Part model, mm, in its own coordinate system. A direction names the side the tool comes from. Round coordinates to 2 decimals unless told otherwise and drop trailing zeros. Loops run counter-clockwise (first coordinate to the right, second up) from the corner with the lowest first, then second, coordinate; pieces in that order, holes last. Notation, with made-up numbers: M 80.5,-12.5 L 126.5,-12.5 A35 ccw 126.5,20.5 Z; hole C 84.25,45.5 d11. An arc over 180 degrees is marked long. Put each result on its own line as item: value. Start each with the question number.
1) Pull direction Z, two halves, no side cores. Call faces 4 (the flat face through (99, 5.08, 80)), 5 (the cylindrical face through (-14.32, 2.5, 157.6)), 6 (the cylindrical face through (-5.091, 2.504, 170.157)): +Z half, -Z half, draft (parallel to the pull), parting line (faces both ways), or undercut.
2) Drop flat-ended pins along their axis: pin 1 Ø5.5 at (x, z) = (21.7, 156.88) entering from +Y; pin 2 Ø1.5 at (x, y) = (164.5, 2) entering from +Z; pin 3 Ø2 at (x, y) = (-14.5, 2) entering from +Z; pin 4 Ø2 at (x, y) = (5.5, 3.5) entering from -Z. Give the stop position or say it passes through.
3) Probe line 1 along X through (y, z) = (0.75, 49); line 2 along X through (y, z) = (3.85, 107.5); line 3 along Z through (x, y) = (-3.5, 2.3). List the from-to ranges inside material, lowest first.
4) Slice it at C-C on z = 107.5. Give the cut face in (x, y).
5) Which spindle directions (+Z, -Z, +X, -X, +Y, -Y) get a long thin tool onto all of the face, cutting with end or side? Do faces 1 (the cylindrical face through (211.089, 2.576, 141.796)), 2 (the flat face through (209.902, 2.576, 24.426)), 3 (the flat face through (69.827, 2.576, 71.224)). Say none if no direction does.
6) Slice it at D-D on x = 148. Give the cut face in (y, z).
7) Slice it at A-A on x = 180. Give the cut face in (y, z), then the cut area to 3 significant figures.
8) Slice it at B-B on z = 54.5. Give the cut face in (x, y).
```python
from build123d import *

# Parameters (mm, degrees)
SKETCH3_R           = 2.5
SKETCH3_R_2         = 52.3875
SKETCH3_R_3         = 3.3
SKETCH3_R_4         = 4.5
SKETCH3_R_5         = 27.4955
SKETCH3_R_6         = 3.300000004
BOSS_EXTRUDE1_DEPTH = 5.08
CUT_EXTRUDE1_REACH  = 321.397
CUT_EXTRUDE2_REACH  = 321.397
CUT_EXTRUDE4_REACH  = 321.397
CUT_EXTRUDE5_REACH  = 321.397
CUT_EXTRUDE6_REACH  = 321.397
FILLET1_R           = 6.604


with BuildPart() as part:
    # Sketch3 → Boss-Extrude1 (new body)
    with BuildSketch(Plane(origin=(0, 0, 0), x_dir=(-1, 0, 0), z_dir=(0, 1, 0))):
        with BuildLine():
            Line((-47.164225852, 28.786858925), (1.714987837, 81.055723289))
            ThreePointArc((1.714987837, 81.055723289), (46.941307752, 112.338258021), (29.825562347, 164.597881552))
            ThreePointArc((29.825562347, 164.597881552), (28.145398332, 165.051242365), (26.567761736, 164.316701751))
            Line((26.567761736, 164.316701751), (21.302878118, 159.051818133))
            ThreePointArc((21.302878118, 159.051818133), (14.21924173, 157.642795249), (10.20668404, 163.648012211))
            Line((10.20668404, 163.648012211), (10.20668404, 170.220745001))
            ThreePointArc((10.20668404, 170.220745001), (9.549518747, 171.925600851), (7.91807501, 172.748273949))
            ThreePointArc((7.91807501, 172.748273949), (3.367898451, 172.974), (-1.182278109, 172.748273949))
            ThreePointArc((-1.182278109, 172.748273949), (-2.813721846, 171.925600851), (-3.470887139, 170.220745001))
            Line((-3.470887139, 170.220745001), (-3.470887139, 163.648012211))
            ThreePointArc((-3.470887139, 163.648012211), (-9.970887139, 157.148012211), (-16.470887139, 163.648012211))
            Line((-16.470887139, 163.648012211), (-16.470887139, 164.225022653))
            ThreePointArc((-16.470887139, 164.225022653), (-17.760387302, 166.435870942), (-20.319588051, 166.401924563))
            Line((-20.319588051, 166.401924563), (-168.403592651, 158.863977372))
            Line((-168.403592651, 158.863977372), (-265.178957518, 163.648012211))
            Line((-265.178957518, 163.648012211), (-268.446360693, 19.778758396))
            ThreePointArc((-268.446360693, 19.778758396), (-262.000922025, 10.329558641), (-251.128758127, 13.883022842))
            Line((-251.128758127, 13.883022842), (-65.147106167, 22.945506915))
            ThreePointArc((-65.147106167, 22.945506915), (-52.854167936, 15.702363891), (-47.164225852, 28.786858925))
        make_face()
        with Locations(Location((-168.403592651, 39.801477371, 0), (0, 0, 90))):
            Circle(SKETCH3_R, mode=Mode.SUBTRACT)
        with Locations(Location((-225.553592651, 96.951477371, 0), (0, 0, 90))):
            Circle(SKETCH3_R, mode=Mode.SUBTRACT)
        with Locations(Location((-168.403592651, 96.951477372, 0), (0, 0, 90))):
            Circle(SKETCH3_R_2, mode=Mode.SUBTRACT)
        with Locations(Location((-111.253592651, 96.951477371, 0), (0, 0, 90))):
            Circle(SKETCH3_R, mode=Mode.SUBTRACT)
        with Locations(Location((-168.403592651, 154.101477371, 0), (0, 0, 90))):
            Circle(SKETCH3_R, mode=Mode.SUBTRACT)
        with Locations(Location((-55.796807523, 24.761419982, 0), (0, 0, 90))):
            Circle(SKETCH3_R_3, mode=Mode.SUBTRACT)
        with Locations(Location((28.436615228, 156.875733282, 0), (0, 0, 90))):
            Circle(SKETCH3_R_4, mode=Mode.SUBTRACT)
        with Locations(Location((-9.970887139, 90.351987789, 0), (0, 0, 90))):
            Circle(SKETCH3_R_4, mode=Mode.SUBTRACT)
        with Locations(Location((16.70668404, 90.351987789, 0), (0, 0, 90))):
            Circle(SKETCH3_R_4, mode=Mode.SUBTRACT)
        with Locations(Location((-30.407092297, 107.5, 0), (0, 0, 90))):
            Circle(SKETCH3_R_4, mode=Mode.SUBTRACT)
        with Locations(Location((37.142889198, 107.5, 0), (0, 0, 90))):
            Circle(SKETCH3_R_4, mode=Mode.SUBTRACT)
        with Locations(Location((3.367898451, 127, 0), (0, 0, 90))):
            Circle(SKETCH3_R_5, mode=Mode.SUBTRACT)
        with Locations(Location((-35.039603917, 133.772278929, 0), (0, 0, 90))):
            Circle(SKETCH3_R_4, mode=Mode.SUBTRACT)
        with Locations(Location((41.775400818, 133.772278929, 0), (0, 0, 90))):
            Circle(SKETCH3_R_4, mode=Mode.SUBTRACT)
        with Locations(Location((-21.700818327, 156.875733282, 0), (0, 0, 90))):
            Circle(SKETCH3_R_4, mode=Mode.SUBTRACT)
        with Locations(Location((3.367898451, 166, 0), (0, 0, 90))):
            Circle(SKETCH3_R_4, mode=Mode.SUBTRACT)
        with Locations(Location((-258.931181349, 19.346338398, 0), (0, 0, 90))):
            Circle(SKETCH3_R_6, mode=Mode.SUBTRACT)
    extrude(amount=BOSS_EXTRUDE1_DEPTH)

    # Sketch9 → Cut-Extrude1 (cut, up to next)
    with BuildSketch(Plane(origin=(0, 5.08, 0), x_dir=(1, 0, 0), z_dir=(0, 1, 0)), mode=Mode.PRIVATE) as cut_extrude1_sk1:
        with BuildLine():
            Line((230.316092651, -96.951477372), (268.099780231, -35.039278689))
            Line((268.099780231, -35.039278689), (265.178957518, -163.648012211))
            Line((265.178957518, -163.648012211), (168.403592651, -158.863977372))
            ThreePointArc((168.403592651, -158.863977372), (212.182341242, -140.730225962), (230.316092651, -96.951477372))
        make_face()
    cut_extrude1_tool1 = extrude(cut_extrude1_sk1.sketch, amount=-CUT_EXTRUDE1_REACH, mode=Mode.PRIVATE) & part.part
    # Sketch9 → Cut-Extrude1 (cut, up to next)
    with BuildSketch(Plane(origin=(0, 5.08, 0), x_dir=(1, 0, 0), z_dir=(0, 1, 0)), mode=Mode.PRIVATE) as cut_extrude1_sk2:
        Polygon((251.128758127, -13.883022842), (168.403592651, -35.038977372), (65.147106167, -22.945506915), align=None)
    cut_extrude1_tool2 = extrude(cut_extrude1_sk2.sketch, amount=-CUT_EXTRUDE1_REACH, mode=Mode.PRIVATE) & part.part
    add(cut_extrude1_tool1.solids().sort_by_distance((243.183286, 5.08, 119.496807))[0], mode=Mode.SUBTRACT)
    add(cut_extrude1_tool2.solids().sort_by_distance((161.559819, 5.08, 23.955836))[0], mode=Mode.SUBTRACT)

    # Sketch10 → Cut-Extrude2 (cut, up to next)
    with BuildSketch(Plane(origin=(0, 5.08, 0), x_dir=(1, 0, 0), z_dir=(0, 1, 0)), mode=Mode.PRIVATE) as cut_extrude2_sk1:
        with BuildLine():
            Line((126.96440839, -43.634475041), (57.261500394, -35.47082269))
            ThreePointArc((57.261500394, -35.47082269), (55.779720918, -35.645410279), (54.535819255, -36.469339824))
            Line((54.535819255, -36.469339824), (31.105609691, -61.52437556))
            ThreePointArc((31.105609691, -61.52437556), (30.434157188, -64.830429418), (33.082361116, -66.920371173))
            Line((33.082361116, -66.920371173), (107.615117732, -75.649698704))
            ThreePointArc((107.615117732, -75.649698704), (109.679489327, -75.212634657), (111.057673768, -73.614741447))
            ThreePointArc((111.057673768, -73.614741447), (118.395945624, -60.449519959), (128.697936364, -49.447598425))
            ThreePointArc((128.697936364, -49.447598425), (129.74459894, -45.970434966), (126.96440839, -43.634475041))
        make_face()
    cut_extrude2_tool1 = extrude(cut_extrude2_sk1.sketch, amount=-CUT_EXTRUDE2_REACH, mode=Mode.PRIVATE) & part.part
    add(cut_extrude2_tool1.solids().sort_by_distance((80.43858, 5.08, 55.50935))[0], mode=Mode.SUBTRACT)

    # Sketch12 → Cut-Extrude4 (cut, up to next)
    with BuildSketch(Plane(origin=(0, 5.08, 0), x_dir=(1, 0, 0), z_dir=(0, 1, 0)), mode=Mode.PRIVATE) as cut_extrude4_sk1:
        with BuildLine():
            Line((249.691658934, -31.738357521), (242.839914491, -63.203787175))
            ThreePointArc((242.839914491, -63.203787175), (240.68572501, -65.624297911), (237.499041194, -65.037398593))
            Line((237.499041194, -65.037398593), (210.225893969, -42.298994776))
            ThreePointArc((210.225893969, -42.298994776), (209.119626938, -39.034817578), (211.522257638, -36.56377625))
            Line((211.522257638, -36.56377625), (245.647149306, -27.836750413))
            ThreePointArc((245.647149306, -27.836750413), (248.757771926, -28.659322972), (249.691658934, -31.738357521))
        make_face()
    cut_extrude4_tool1 = extrude(cut_extrude4_sk1.sketch, amount=-CUT_EXTRUDE4_REACH, mode=Mode.PRIVATE) & part.part
    add(cut_extrude4_tool1.solids().sort_by_distance((232.663577, 5.08, 44.411136))[0], mode=Mode.SUBTRACT)

    # Sketch13 → Cut-Extrude5 (cut, up to next)
    with BuildSketch(Plane(origin=(0, 5.08, 0), x_dir=(1, 0, 0), z_dir=(0, 1, 0)), mode=Mode.PRIVATE) as cut_extrude5_sk1:
        with BuildLine():
            Line((103.453694718, -97.126401755), (36.43287071, -100.986145044))
            ThreePointArc((36.43287071, -100.986145044), (34.842208875, -100.679745253), (33.588682349, -99.653705706))
            ThreePointArc((33.588682349, -99.653705706), (30.860299189, -96.307343511), (27.830020313, -93.231693249))
            ThreePointArc((27.830020313, -93.231693249), (26.949082998, -89.730069681), (29.800859551, -87.515393937))
            Line((29.800859551, -87.515393937), (104.077509501, -81.423867894))
            ThreePointArc((104.077509501, -81.423867894), (106.803706724, -82.508060349), (107.590756045, -85.334396836))
            ThreePointArc((107.590756045, -85.334396836), (106.923967125, -89.643036953), (106.562061414, -93.987920308))
            ThreePointArc((106.562061414, -93.987920308), (105.609941649, -96.153447619), (103.453694718, -97.126401755))
        make_face()
    cut_extrude5_tool1 = extrude(cut_extrude5_sk1.sketch, amount=-CUT_EXTRUDE5_REACH, mode=Mode.PRIVATE) & part.part
    add(cut_extrude5_tool1.solids().sort_by_distance((69.06396, 5.08, 91.55919))[0], mode=Mode.SUBTRACT)

    # Sketch11 → Cut-Extrude6 (cut, up to next)
    with BuildSketch(Plane(origin=(0, 5.08, 0), x_dir=(1, 0, 0), z_dir=(0, 1, 0)), mode=Mode.PRIVATE) as cut_extrude6_sk1:
        with BuildLine():
            ThreePointArc((109.17784979, -114.992237854), (107.925725235, -113.25846106), (105.873806466, -112.655611792))
            Line((105.873806466, -112.655611792), (45.047435633, -115.33547257))
            ThreePointArc((45.047435633, -115.33547257), (42.621254202, -116.562921091), (41.938707081, -119.194862511))
            ThreePointArc((41.938707081, -119.194862511), (42.605357512, -126.738442657), (42.024583396, -134.289119823))
            ThreePointArc((42.024583396, -134.289119823), (40.637406634, -140.309462815), (38.45555618, -146.089455697))
            ThreePointArc((38.45555618, -146.089455697), (38.718980125, -149.302538125), (41.594710316, -150.759750098))
            Line((41.594710316, -150.759750098), (123.487203332, -147.402375423))
            ThreePointArc((123.487203332, -147.402375423), (126.441313333, -145.268908214), (125.633039875, -141.715720596))
            ThreePointArc((125.633039875, -141.715720596), (115.684078111, -129.413924027), (109.17784979, -114.992237854))
        make_face()
    cut_extrude6_tool1 = extrude(cut_extrude6_sk1.sketch, amount=-CUT_EXTRUDE6_REACH, mode=Mode.PRIVATE) & part.part
    add(cut_extrude6_tool1.solids().sort_by_distance((79.387948, 5.08, 132.50433))[0], mode=Mode.SUBTRACT)

    # Fillet1
    fillet1_edges = [part.edges().sort_by_distance(p)[0] for p in [
        (230.316092651, 2.54, 96.951477372),
        (168.403592651, 2.54, 35.038977372),
        (-1.714987837, 2.54, 81.055723289),
        (47.164225852, 2.54, 28.786858925),
        (65.147106167, 2.54, 22.945506915),
        (251.128758127, 2.54, 13.883022842),
    ]]
    fillet(fillet1_edges, radius=FILLET1_R)


solid = part.part
```
Recorded:
1. face 4: draft
1. face 5: +Z half
1. face 6: undercut
2. pin 1: passes through
2. pin 2: stops at z = 159.1
2. pin 3: stops at z = 157.99
2. pin 4: stops at z = 72.27
3. line 1: x = 28.26 to 42.82, 129.14 to 147.31, 189.5 to 218.26, 245.93 to 259.58
3. line 2: x = -45 to -41.64, -32.64 to -22.75, 16.02 to 25.91, 34.91 to 117.09, 219.72 to 229.41
3. line 3: z = 80.95 to 99.5, 154.5 to 161.5, 170.5 to 172.97
4. outline: M -45,0 L -41.64,0 L -41.64,5.08 L -45,5.08 Z; M -32.64,0 L -22.75,0 L -22.75,5.08 L -32.64,5.08 Z; M 16.02,0 L 25.91,0 L 25.91,5.08 L 16.02,5.08 Z; M 34.91,0 L 117.09,0 L 117.09,5.08 L 34.91,5.08 Z; M 219.72,0 L 229.41,0 L 229.41,5.08 L 219.72,5.08 Z
5. face 1: +Z, +X, +Y, -Y
5. face 2: -Z, +Y, -Y
5. face 3: +Y, -Y
6. outline: M 0,32.65 L 5.08,32.65 L 5.08,48.7 L 0,48.7 Z; M 0,145.2 L 5.08,145.2 L 5.08,159.9 L 0,159.9 Z
7. outline: M 0,32.07 L 5.08,32.07 L 5.08,45.86 L 0,45.86 Z; M 0,148.04 L 5.08,148.04 L 5.08,157.77 L 0,157.77 Z
7. area: 119 mm2
8. outline: M 23.12,0 L 37.67,0 L 37.67,5.08 L 23.12,5.08 Z; M 123.34,0 L 137.71,0 L 137.71,5.08 L 123.34,5.08 Z; M 199.1,0 L 224.86,0 L 224.86,5.08 L 199.1,5.08 Z; M 244.74,0 L 256.22,0 L 256.22,5.08 L 244.74,5.08 Z
